```python
from build123d import *

# Parameters (mm, degrees)
SKETCH1_W           = 17
SKETCH1_H           = 30
BOSS_EXTRUDE1_DEPTH = 3
SKETCH2_W           = 3
SKETCH2_H           = 5
CUT_EXTRUDE1_DEPTH  = 3
SKETCH3_R           = 1.5
CUT_EXTRUDE2_DEPTH  = 3
FILLET1_R           = 3


with BuildPart() as part:
    # Sketch1 → Boss-Extrude1 (new body)
    with BuildSketch(Plane(origin=(0, 0, 0), x_dir=(1, 0, 0), z_dir=(0, 1, 0))):
        Rectangle(SKETCH1_W, SKETCH1_H)
    extrude(amount=BOSS_EXTRUDE1_DEPTH)

    # Sketch2 → Cut-Extrude1 (cut)
    with BuildSketch(Plane(origin=(0, 3, 0), x_dir=(1, 0, 0), z_dir=(0, 1, 0))):
        with Locations((7, 10)):
            Rectangle(SKETCH2_W, SKETCH2_H)
        with Locations((7, 0)):
            Rectangle(SKETCH2_W, SKETCH2_H)
        with Locations((7, -10)):
            Rectangle(SKETCH2_W, SKETCH2_H)
    extrude(amount=-CUT_EXTRUDE1_DEPTH, mode=Mode.SUBTRACT)

    # Sketch3 → Cut-Extrude2 (cut)
    with BuildSketch(Plane(origin=(0, 3, 0), x_dir=(1, 0, 0), z_dir=(0, 1, 0))):
        with Locations(Location((-4.5, 10, 0), (0, 0, 270))):
            Circle(SKETCH3_R)
        with Locations(Location((-4.5, -10, 0), (0, 0, 270))):
            Circle(SKETCH3_R)
    extrude(amount=-CUT_EXTRUDE2_DEPTH, mode=Mode.SUBTRACT)

    # Fillet1
    fillet1_edges = [part.edges().sort_by_distance(p)[0] for p in [
        (-8.5, 1.5, 15),
        (-8.5, 1.5, -15),
    ]]
    fillet(fillet1_edges, radius=FILLET1_R)


solid = part.part
```
CAD build for the part. Positions are in the model's coordinates, mm. A direction names the side the tool comes from. Round coordinates to 2 decimals unless told otherwise and drop trailing zeros. Order: outer loops, then holes, each group sorted by start corner. A loop starts at its lowest first (then second) coordinate and runs counter-clockwise, first axis right, second up. Notation, with made-up numbers: (5.25, 1) - (64.25, 1) arc R12 cw to (64.25, 7) - close; hole circle Ø5 at (70.5, -12). An arc over 180 degrees is marked (long way). Use CSV: the item, a comma, the result in double quotes. Start each with the question number.
1) Two-plate mould, pull along Z, no slides. Class faces 1 (the flat face through (7, 2, -2.5)), 2 (the flat face through (8.5, 1, 5)), 3 (the cylindrical face through (-7.64, 1.52, 14.1)): pulls with the +Z half, pulls with the -Z half, needs draft (parallel to the pull), parting line crosses it, or undercut.
2) Wall check: L1, parallel to Z at x = 7.5, y = 2.7; L2, parallel to X at y = 1.2, z = 10; L3, parallel to X at y = 2, z = 0.25. Give the ranges that are in metal, low to high. Write a range as [from, to].
3) Tool access for faces 4 (the cylindrical face through (-4.43, 1.52, 8.5)), 5 (the flat face through (7, 2, -7.5)): list every direction of +Z, -Z, +X, -X, +Y, -Y with a clear straight run to the whole face (end or side of a thin tool).
4) Saw through at D-D (y = 0.5). List the corners of the cut face in (x, z).
5) Saw through at A-A (x = -4.5). List the corners of the cut face in (y, z), and give its area (3 significant figures).
6) Pin check, flat tip, straight feed: pin 1 Ø1.5 at (y, z) = (1.5, -9.5) entering from +X. Stop position of the tip, or through.
7) Saw through at B-B (x = 7). List the corners of the cut face in (y, z), and give its area (3 significant figures).
8) Saw through at C-C (z = -10). List the corners of the cut face in (x, y), and give its area (3 significant figures).
Values follow:
1,face 1,"undercut"
1,face 2,"needs draft"
1,face 3,"pulls with the +Z half"
2,L1,"z = [-15, -12.5], [-7.5, -2.5], [2.5, 7.5], [12.5, 15]"
2,L2,"x = [-8.5, -6], [-3, 5.5]"
2,L3,"x = [-8.5, 5.5]"
3,face 4,"+Y, -Y"
3,face 5,"+X, +Y, -Y"
4,outline,"(-8.5, -12) arc R3 ccw to (-5.5, -15) - (8.5, -15) - (8.5, -12.5) - (5.5, -12.5) - (5.5, -7.5) - (8.5, -7.5) - (8.5, -2.5) - (5.5, -2.5) - (5.5, 2.5) - (8.5, 2.5) - (8.5, 7.5) - (5.5, 7.5) - (5.5, 12.5) - (8.5, 12.5) - (8.5, 15) - (-5.5, 15) arc R3 ccw to (-8.5, 12) - close; hole circle Ø3 at (-4.5, -10); hole circle Ø3 at (-4.5, 10)"
5,outline,"(0, -15) - (3, -15) - (3, -11.5) - (0, -11.5) - close; (0, -8.5) - (3, -8.5) - (3, 8.5) - (0, 8.5) - close; (0, 11.5) - (3, 11.5) - (3, 15) - (0, 15) - close"
5,area,"72.0 mm2"
6,pin 1,"stops at x = 5.5"
7,outline,"(0, -15) - (3, -15) - (3, -12.5) - (0, -12.5) - close; (0, -7.5) - (3, -7.5) - (3, -2.5) - (0, -2.5) - close; (0, 2.5) - (3, 2.5) - (3, 7.5) - (0, 7.5) - close; (0, 12.5) - (3, 12.5) - (3, 15) - (0, 15) - close"
7,area,"45.0 mm2"
8,outline,"(-8.5, 0) - (-6, 0) - (-6, 3) - (-8.5, 3) - close; (-3, 0) - (5.5, 0) - (5.5, 3) - (-3, 3) - close"
8,area,"33.0 mm2"
